```python
from build123d import *

# Parameters (mm, degrees)
SKETCH1_R                           = 65
BOSS_EXTRUDE1_DEPTH                 = 5
CUT_EXTRUDE2_START                  = -25
CUT_EXTRUDE2_DEPTH                  = 25
FILLET2_R                           = 12
SKETCH9_R                           = 12.5
BOSS_EXTRUDE4_DEPTH                 = 30
SKETCH10_R                          = 4.95
CUT_EXTRUDE3_DEPTH                  = 97.34882957
SKETCH11_W                          = 5
SKETCH11_H                          = 5
CUT_EXTRUDE4_DEPTH                  = 97.34882957
F_1_0MM_DOWEL_HOLE3_D               = 2.8
F_1_0MM_DOWEL_HOLE3_DEPTH           = 33.158795133
F_1_0MM_DOWEL_HOLE3_TIP             = 0.841204867
F_1_0MM_DOWEL_HOLE3_ON_FACE_2_D     = 2.8
F_1_0MM_DOWEL_HOLE3_ON_FACE_2_DEPTH = 33.158795133
F_1_0MM_DOWEL_HOLE3_ON_FACE_2_TIP   = 0.841204867
BOSS_EXTRUDE5_DEPTH                 = 4
BOSS_EXTRUDE5_DEPTH_BACK            = 5
SKETCH13_R                          = 37.8
F_1_0MM_DOWEL_HOLE4_D               = 9.2
F_1_0MM_DOWEL_HOLE4_DEPTH           = 31.236041152
F_1_0MM_DOWEL_HOLE4_TIP             = 2.763958848
FILLET4_R                           = 15


with BuildPart() as part:
    # Sketch1 → Boss-Extrude1 (new body)
    with BuildSketch(Plane.XY):
        Circle(SKETCH1_R)
    extrude(amount=BOSS_EXTRUDE1_DEPTH)

    # Sketch6 → Cut-Extrude2 (cut)
    with BuildSketch(Plane.XY.offset(5).offset(CUT_EXTRUDE2_START)):
        with BuildLine():
            ThreePointArc((0, 65), (-47.923026893, 43.913363495), (-64.752655376, -5.665123279))
            ThreePointArc((-64.752655376, -5.665123279), (-20.242011997, 18.548386617), (0, 65))
        make_face()
        with BuildLine():
            ThreePointArc((37.282468363, -53.244882879), (-5.942368011, -26.804289921), (-56.291651246, -32.5))
            ThreePointArc((-56.291651246, -32.5), (-14.068574906, -63.459240463), (37.282468363, -53.244882879))
        make_face()
        with BuildLine():
            ThreePointArc((56.291651246, -32.5), (61.991601799, 19.545876968), (27.470187013, 58.910006157))
            ThreePointArc((27.470187013, 58.910006157), (26.184380008, 8.255903304), (56.291651246, -32.5))
        make_face()
    extrude(amount=CUT_EXTRUDE2_DEPTH, mode=Mode.SUBTRACT)

    # Fillet2
    fillet2_edges = [part.edges().sort_by_distance(p)[0] for p in [
        (27.470187013, 58.910006157, 2.5),
        (56.291651246, -32.5, 2.5),
        (-64.752655376, -5.665123279, 2.5),
        (0, 65, 2.5),
        (37.282468363, -53.244882879, 2.5),
        (-56.291651246, -32.5, 2.5),
    ]]
    fillet(fillet2_edges, radius=FILLET2_R)

    # Sketch9 → Boss-Extrude4 (add)
    with BuildSketch(Plane(origin=(0, 0, 0), x_dir=(-1, 0, 0), z_dir=(0, 0, -1))):
        with Locations(Location((0, 0, 0), (0, 0, 180))):
            Circle(SKETCH9_R)
    extrude(amount=BOSS_EXTRUDE4_DEPTH)

    # Sketch10 → Cut-Extrude3 (cut, through all)
    with BuildSketch(Plane(origin=(0, 0, -30), x_dir=(-1, 0, 0), z_dir=(0, 0, -1))):
        Circle(SKETCH10_R)
    extrude(amount=-CUT_EXTRUDE3_DEPTH, mode=Mode.SUBTRACT)

    # Sketch11 → Cut-Extrude4 (cut, through all)
    with BuildSketch(Plane(origin=(0, 0, -30), x_dir=(-1, 0, 0), z_dir=(0, 0, -1))):
        with Locations((0, 4.95)):
            Rectangle(SKETCH11_W, SKETCH11_H)
    extrude(amount=-CUT_EXTRUDE4_DEPTH, mode=Mode.SUBTRACT)

    # Ø1.0mm Dowel Hole3
    with Locations(Plane(origin=(0, -12.5, -18.578187756), x_dir=(-1, 0, 0), z_dir=(0, -1, 0))):
        with Locations((0, 0)):
            Hole(F_1_0MM_DOWEL_HOLE3_D / 2, depth=F_1_0MM_DOWEL_HOLE3_DEPTH)
            with Locations((0, 0, -(F_1_0MM_DOWEL_HOLE3_DEPTH + F_1_0MM_DOWEL_HOLE3_TIP / 2))):  # 118° drill point
                Cone(0, F_1_0MM_DOWEL_HOLE3_D / 2, F_1_0MM_DOWEL_HOLE3_TIP, mode=Mode.SUBTRACT)

    # Ø1.0mm Dowel Hole3 on face 2
    with Locations(Plane(origin=(12.447431605, 1.14518402, -23.093887112), x_dir=(-0.091614954639, 0.995794506957, 0), z_dir=(0.995794506957, 0.091614954639, 0))):
        with Locations((0, 0)):
            Hole(F_1_0MM_DOWEL_HOLE3_ON_FACE_2_D / 2, depth=F_1_0MM_DOWEL_HOLE3_ON_FACE_2_DEPTH)
            with Locations((0, 0, -(F_1_0MM_DOWEL_HOLE3_ON_FACE_2_DEPTH + F_1_0MM_DOWEL_HOLE3_ON_FACE_2_TIP / 2))):  # 118° drill point
                Cone(0, F_1_0MM_DOWEL_HOLE3_ON_FACE_2_D / 2, F_1_0MM_DOWEL_HOLE3_ON_FACE_2_TIP, mode=Mode.SUBTRACT)

    # Sketch13 → Boss-Extrude5 (add, two sides: drawn at the far end of the back side and taken through both)
    with BuildSketch(Plane(origin=(0, 0, 0), x_dir=(-1, 0, 0), z_dir=(0, 0, -1)).offset(-BOSS_EXTRUDE5_DEPTH_BACK)):
        Circle(SKETCH13_R)
    extrude(amount=BOSS_EXTRUDE5_DEPTH + BOSS_EXTRUDE5_DEPTH_BACK)

    # Ø1.0mm Dowel Hole4
    with Locations(Plane(origin=(10.821980697, 48.814800356, 0), x_dir=(-1, 0, 0), z_dir=(0, 0, -1))):
        with Locations((0, 0), (59.310094228, -65.476990486), (-26.041886144, -82.594310737)):
            Hole(F_1_0MM_DOWEL_HOLE4_D / 2, depth=F_1_0MM_DOWEL_HOLE4_DEPTH)
            with Locations((0, 0, -(F_1_0MM_DOWEL_HOLE4_DEPTH + F_1_0MM_DOWEL_HOLE4_TIP / 2))):  # 118° drill point
                Cone(0, F_1_0MM_DOWEL_HOLE4_D / 2, F_1_0MM_DOWEL_HOLE4_TIP, mode=Mode.SUBTRACT)

    # Fillet4
    # the kernel refuses this fillet: 15 mm, written as the material it adds along each edge
    with BuildSketch(Plane(origin=(0, 0, -4), x_dir=(1, 0, 0), z_dir=(0, -1, 0))) as fillet4_piece_1_section:
        with BuildLine():
            CenterArc((12.5 + FILLET4_R, -FILLET4_R), FILLET4_R, 90, 90)
            Line((12.5, -FILLET4_R), (12.5, 0))
            Line((12.5, 0), (12.5 + FILLET4_R, 0))
        make_face()
    fillet4_piece_1 = revolve(axis=Axis((0, 0, -4), (0, 0, 1)), mode=Mode.PRIVATE)
    fillet4_piece_1 = fillet4_piece_1 - Plane(origin=(0, 0, -18.578187756), x_dir=(1, 0, 0), z_dir=(0, 1, 0)) * Cylinder(1.4, 110, mode=Mode.PRIVATE)
    add(fillet4_piece_1)


solid = part.part
```
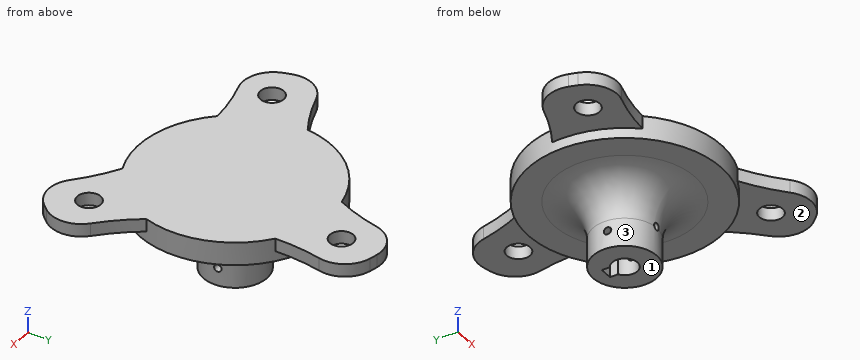
Geometry check sheet. Reference: the model listing, model coordinates, mm. Face numbers are marked on the shaded views. A direction names the side the tool comes from. Coordinates: 2 decimals unless noted, no trailing zeros. Loops run counter-clockwise (first coordinate to the right, second up) from the corner with the lowest first, then second, coordinate; pieces in that order, holes last. Notation, with made-up numbers: (-27, 56) - (2, 56) arc R21 ccw to (2, 89) - close; hole circle Ø10 at (43.5, 39). An arc over 180 degrees is marked (long way). One line per item, written item: value. Start each with the question number.
(1) Cross-section at C-C on z = -9.5. Enter the section's corners in (x, y), plus the area to 3 significant figures.
(2) Depth check by flat-ended pin: P1, Ø9.5, axis at x = 10.5, y = 47.5, coming from the -Z side; P2, Ø5.5, axis at x = -0.5, z = -21.5, coming from the -Y side; P3, Ø3.5, axis at x = 0, z = -18.58, coming from the -Y side; P4, Ø2, axis at x = 0, z = -18.58, coming from the -Y side. Enter the tip coordinate at first touch or a pass-through.
(3) Tool access check on the marked faces 1, 2 and 3. Record the directions out of +Z, -Z, +X, -X, +Y, -Y that give a thin tool (end or side, any length) a straight path to the whole face; none if there is none.
(4) Cross-section at A-A on x = -30. Enter the section's corners in (y, z).
(5) Material ranges on line 1 (Y direction, x = -1, z = -6.5); line 2 (Z direction, x = -7, y = 36); line 3 (Y direction, x = 0, z = -12), recorded low to high. Write a range as [from, to].
(6) Cross-section at B-B on z = -2. Enter the section's corners in (x, y).
(7) Cross-section at D-D on x = 0. Count the separate pieces of the cut face and the enclosed holes in it, plus the area to 3 significant figures.
Results below:
1. outline: circle Ø31.78 at (0, 0); hole (-2.5, 4.27) arc R4.95 ccw (long way) to (2.5, 4.27) - (2.5, 7.45) - (-2.5, 7.45) - close
1. area: 703 mm2
2. P1: stops at z = 0
2. P2: stops at y = -12.5
2. P3: stops at y = -12.66
2. P4: passes through
3. face 1: -Z, +X, -X, +Y, -Y
3. face 2: -Z, +X, -Y
3. face 3: -Z
4. outline: (-25.29, 0) - (-23, 0) - (-23, -4) - (23, -4) - (23, 5) - (-25.29, 5) - close
5. line 1: y = [-19.18, -4.85], [7.45, 19.18]
5. line 2: z = [-4, 5]
5. line 3: y = [-14.23, -4.95], [7.45, 14.23]
6. outline: circle Ø75.6 at (0, 0)
7. separate pieces: 3
7. enclosed holes: 0
7. area: 1,170 mm2
